Source: CAD feature listing. Evaluate the final solid. Frame: model axes, mm. Coordinates: 2 decimals unless noted, no trailing zeros. Loops run counter-clockwise (first coordinate to the right, second up) from the corner with the lowest first, then second, coordinate; pieces in that order, holes last. Notation, with made-up numbers: (54.25, 17.25) -> (101.25, 17.25) arc R26 ccw to (101.25, 46.25) -> close; hole circle Ø3 at (0.25, -16). An arc over 180 degrees is marked (long way). Answer as CSV lines item,"result".
from build123d import *

# Parameters (mm, degrees)
SKETCH1_W                 = 88
SKETCH1_H                 = 211
BOSS_EXTRUDE1_DEPTH       = 2
CUT_EXTRUDE2_DEPTH        = 2
SKETCH4_R                 = 5
CUT_EXTRUDE3_DEPTH        = 3
FILLET2_R                 = 3
SKETCH23_W                = 2
SKETCH23_H                = 211
SKETCH23_W_2              = 2.150374681
CUT_EXTRUDE5_DEPTH        = 10
SKETCH29_W                = 5.911493913
SKETCH29_H                = 211
SKETCH29_W_2              = 4.036537762
CUT_EXTRUDE10_DEPTH       = 2
M3X0_5_TAPPED_HOLE1_D     = 2.5
M3X0_5_TAPPED_HOLE1_DEPTH = 10
M3X0_5_TAPPED_HOLE1_TIP   = 0.751075774


with BuildPart() as part:
    # Sketch1 → Boss-Extrude1 (new body)
    with BuildSketch(Plane.XY):
        with Locations((44, 105.5)):
            Rectangle(SKETCH1_W, SKETCH1_H)
    extrude(amount=BOSS_EXTRUDE1_DEPTH)

    # Sketch3 → Cut-Extrude2 (cut)
    with BuildSketch(Plane.XY.offset(2)):
        Polygon((73, 133.88804004), (50, 147.167096231), (50, 115.5), (73, 115.5), align=None)
        Polygon((38, 115.5), (38, 147.167096231), (15, 133.88804004), (15, 115.5), align=None)
        Polygon((15, 143.125644347), (36, 155.25), (15, 167.374355653), align=None)
        Polygon((73, 143.125644347), (73, 167.374355653), (52, 155.25), align=None)
        Polygon((73, 196), (50, 196), (50, 163.332903769), (73, 176.61195996), align=None)
        Polygon((38, 163.332903769), (38, 196), (15, 196), (15, 176.61195996), align=None)
    cut_extrude2 = extrude(amount=-CUT_EXTRUDE2_DEPTH, mode=Mode.SUBTRACT)

    # Sketch4 → Cut-Extrude3 (cut, through all)
    with BuildSketch(Plane.XY.offset(2)):
        with Locations((44, 155.25)):
            Circle(SKETCH4_R)
    cut_extrude3 = extrude(amount=-CUT_EXTRUDE3_DEPTH, mode=Mode.SUBTRACT)

    # Mirror2: Cut-Extrude2, Cut-Extrude3 across plane
    add(cut_extrude2.mirror(Plane.ZX.offset(105.5)), mode=Mode.SUBTRACT)
    add(cut_extrude3.mirror(Plane.ZX.offset(105.5)), mode=Mode.SUBTRACT)

    # Fillet2
    fillet2_edges = [part.edges().sort_by_distance(p)[0] for p in [
        (36, 55.75, 1),
        (15, 43.625644347, 1),
        (15, 67.874355653, 1),
        (38, 95.5, 1),
        (38, 63.832903769, 1),
        (15, 77.11195996, 1),
        (15, 95.5, 1),
        (73, 15, 1),
        (50, 15, 1),
        (50, 47.667096231, 1),
        (73, 34.38804004, 1),
        (73, 43.625644347, 1),
        (52, 55.75, 1),
        (73, 67.874355653, 1),
        (15, 15, 1),
        (15, 34.38804004, 1),
        (38, 47.667096231, 1),
        (38, 15, 1),
        (73, 77.11195996, 1),
        (50, 63.832903769, 1),
        (50, 95.5, 1),
        (73, 95.5, 1),
        (15, 167.374355653, 1),
        (36, 155.25, 1),
        (15, 143.125644347, 1),
        (38, 147.167096231, 1),
        (38, 115.5, 1),
        (15, 115.5, 1),
        (15, 133.88804004, 1),
        (50, 196, 1),
        (73, 196, 1),
        (73, 176.61195996, 1),
        (50, 163.332903769, 1),
        (52, 155.25, 1),
        (73, 167.374355653, 1),
        (73, 143.125644347, 1),
        (15, 176.61195996, 1),
        (15, 196, 1),
        (38, 196, 1),
        (38, 163.332903769, 1),
        (50, 147.167096231, 1),
        (73, 133.88804004, 1),
        (73, 115.5, 1),
        (50, 115.5, 1),
    ]]
    fillet(fillet2_edges, radius=FILLET2_R)

    # Sketch23 → Cut-Extrude5 (cut)
    with BuildSketch(Plane.XY.offset(2)):
        with Locations((87, 105.5)):
            Rectangle(SKETCH23_W, SKETCH23_H)
        with Locations((1.075187341, 105.5)):
            Rectangle(SKETCH23_W_2, SKETCH23_H)
    extrude(amount=-CUT_EXTRUDE5_DEPTH, mode=Mode.SUBTRACT)

    # Sketch29 → Cut-Extrude10 (cut)
    with BuildSketch(Plane(origin=(0, 0, 0), x_dir=(-1, 0, 0), z_dir=(0, 0, -1))):
        with Locations((-1.044253043, 105.5)):
            Rectangle(SKETCH29_W, SKETCH29_H)
        with Locations((-86.018268881, 105.5)):
            Rectangle(SKETCH29_W_2, SKETCH29_H)
    extrude(amount=-CUT_EXTRUDE10_DEPTH, mode=Mode.SUBTRACT)

    # M3x0.5 Tapped Hole1
    with Locations(Plane.XY.offset(2)):
        with Locations((9, 186), (9, 139.2), (9, 109.2), (9, 79.2), (9, 59.2), (9, 33.2), (79, 186), (79, 139.2), (79, 109.2), (79, 79.2), (79, 59.2), (79, 33.2), (24, 6), (64, 6), (24, 205), (64, 205), (9, 196), (79, 196), (9, 23), (79, 23)):
            Hole(M3X0_5_TAPPED_HOLE1_D / 2, depth=M3X0_5_TAPPED_HOLE1_DEPTH)
            with Locations((0, 0, -(M3X0_5_TAPPED_HOLE1_DEPTH + M3X0_5_TAPPED_HOLE1_TIP / 2))):  # 118° drill point
                Cone(0, M3X0_5_TAPPED_HOLE1_D / 2, M3X0_5_TAPPED_HOLE1_TIP, mode=Mode.SUBTRACT)


solid = part.part
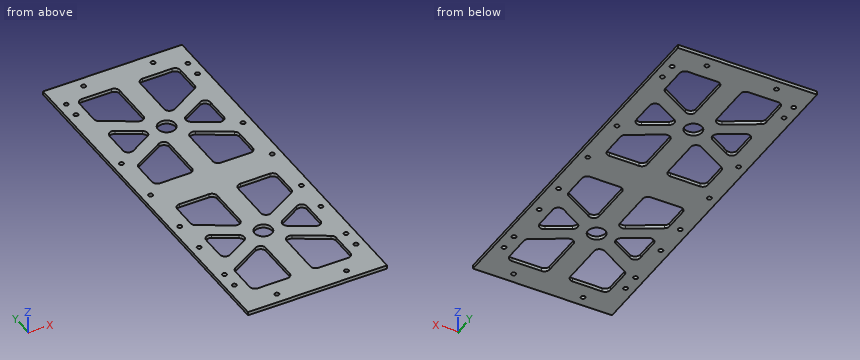
(1) Pin query (flat end, axial travel): pin 1 Ø3 at (x, y) = (79, 139.2) entering from +Z. Return the tip coordinate at first contact, or that it passes through.
Computed values:
pin 1,"z = 2"
(2) Material intervals for L1, parallel to X at y = 123.5, z = 1.3; L2, parallel to X at y = 108.5, z = 0.3, sorted ascending. Write a range as [from, to].
Computed values:
L1,"[4, 15], [38, 50], [73, 84]"
L2,"[4, 7.96], [10.04, 77.96], [80.04, 84]"
(3) Cut plane A-A (x = 44). Return the cut outline in (y, z).
Computed values:
outline,"(0, 0) -> (50.75, 0) -> (50.75, 2) -> (0, 2) -> close; (60.75, 0) -> (150.25, 0) -> (150.25, 2) -> (60.75, 2) -> close; (160.25, 0) -> (211, 0) -> (211, 2) -> (160.25, 2) -> close"
(4) Cut plane B-B (y = 55.75). Return the cut outline in (x, z).
Computed values:
outline,"(4, 0) -> (15, 0) -> (15, 2) -> (4, 2) -> close; (33, 0) -> (39, 0) -> (39, 2) -> (33, 2) -> close; (49, 0) -> (55, 0) -> (55, 2) -> (49, 2) -> close; (73, 0) -> (84, 0) -> (84, 2) -> (73, 2) -> close"
(5) Cut plane C-C (z = 0.45). State how many separate pieces and enclosed holes the cut face has, then the cut area to 3 significant figures.
Computed values:
separate pieces,"1"
enclosed holes,"34"
area,"11,100 mm^2"
